Source: CAD feature listing. Evaluate the final solid. Frame: model axes, mm. Face numbers are marked on the shaded views. A direction names the side the tool comes from. Give positions to 0.01 mm unless a question says otherwise; leave off trailing zeros. Write each loop counter-clockwise with the first axis right and the second up, starting at its lowest first coordinate (ties: lowest second). Pieces come first, ordered by that corner, then holes. Notation, with made-up numbers: M -40,-34 L -3,-34 A10 cw -3,-22 Z; hole C -5,-36 d1. An arc over 180 degrees is marked long. Use CSV: the item, a comma, the result in double quotes. Start each with the question number.
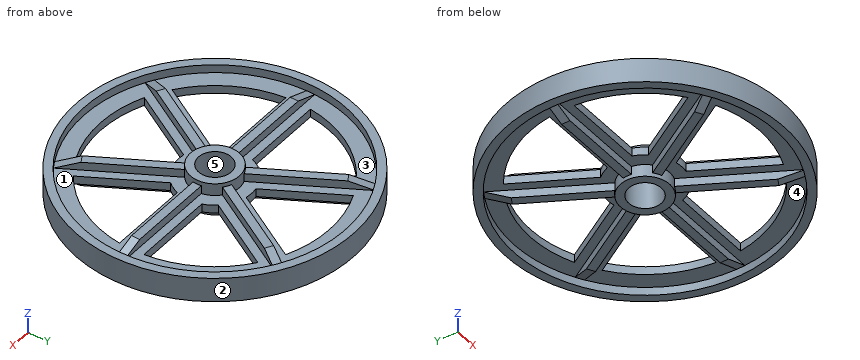
from build123d import *

# Parameters (mm, degrees)
SKETCH1_R           = 15
BOSS_EXTRUDE1_DEPTH = 10
BOSS_EXTRUDE9_DEPTH = 2.5
CIRPATTERN1_COUNT   = 6
CUT_EXTRUDE2_DEPTH  = 5
CIRPATTERN2_COUNT   = 6
SKETCH3_R           = 10
CUT_EXTRUDE3_DEPTH  = 25


with BuildPart() as part:
    # Sketch1 → Boss-Extrude1 (new, symmetric)
    with BuildSketch(Plane.XY):
        Circle(SKETCH1_R)
    extrude(amount=BOSS_EXTRUDE1_DEPTH, both=True)

    # Sketch2 → Revolve1 (revolve)
    with BuildSketch(Plane(origin=(0, 0, 0), x_dir=(0, 0, -1), z_dir=(1, 0, 0)), mode=Mode.PRIVATE) as revolve1_sk:
        Polygon((-2.5, 15), (-2.5, 80), (-7.5, 80), (-7.5, 85), (7.5, 85), (7.5, 80), (2.5, 80), (2.5, 15), align=None)
    revolve(revolve1_sk.sketch.rotate(Axis((0, 0, 0), (0, 0, -1)), 90), axis=Axis((0, 0, 0), (0, 0, -1)))

    # Sketch5 → Boss-Extrude9 (add, symmetric)
    with BuildSketch(Plane(origin=(0, 0, 0), x_dir=(1, 0, 0), z_dir=(0, 1, 0))):
        Polygon((0, -2.5), (-80, -2.5), (-66.262612903, -7.5), (0, -7.5), align=None)
        Polygon((0, 7.5), (-66.262612903, 7.5), (-80, 2.5), (0, 2.5), align=None)
    boss_extrude9 = extrude(amount=BOSS_EXTRUDE9_DEPTH, both=True)

    # CirPattern1: Boss-Extrude9 ×6 about axis
    cirpattern1_axis = Axis((0, 0, 0), (0, 0, 1))
    for i in range(1, CIRPATTERN1_COUNT):
        add(boss_extrude9.rotate(cirpattern1_axis, i * 360 / CIRPATTERN1_COUNT))

    # Sketch6 → Cut-Extrude2 (cut)
    with BuildSketch(Plane.XY.offset(2.5)):
        with BuildLine():
            Line((-17.101792246, 14.621173071), (-41.293717796, 56.522817256))
            ThreePointArc((-41.293717796, 56.522817256), (-60.621778265, 35), (-69.597054535, 7.5))
            Line((-69.597054535, 7.5), (-21.213203436, 7.5))
            ThreePointArc((-21.213203436, 7.5), (-19.485571585, 11.25), (-17.101792246, 14.621173071))
        make_face()
    cut_extrude2 = extrude(amount=-CUT_EXTRUDE2_DEPTH, mode=Mode.SUBTRACT)

    # CirPattern2: Cut-Extrude2 ×6 about axis
    cirpattern2_axis = Axis((0, 0, 0), (0, 0, 1))
    for i in range(1, CIRPATTERN2_COUNT):
        add(cut_extrude2.rotate(cirpattern2_axis, i * 360 / CIRPATTERN2_COUNT), mode=Mode.SUBTRACT)

    # Sketch3 → Cut-Extrude3 (cut)
    with BuildSketch(Plane.XY.offset(10)):
        Circle(SKETCH3_R)
    extrude(amount=-CUT_EXTRUDE3_DEPTH, mode=Mode.SUBTRACT)


solid = part.part
Item 1: Section A-A (x = 0). State how many separate pieces and enclosed holes the cut face has, plus the area to 3 significant figures.
Item 2: Pull-direction query (X, two-part tool) for the marked faces 1 and 2; classes: released by +X, released by -X, zero draft, split by the parting line, or undercut.
Item 3: Section C-C (y = 0). Return the cut outline in (x, z), plus the area to 3 significant figures.
Item 4: Section B-B (z = -5). Return the cut outline in (x, y).
Item 5: Contact query for flat-ended pins moving along their axis: pin 1 Ø6 at (x, z) = (-25, 5.5) entering from -Y; pin 2 Ø2.5 at (x, z) = (49, -6) entering from +Y; pin 3 Ø15 at (x, y) = (-18, -24) entering from +Z. Output: stop coordinate, or through.
Item 6: Section D-D (x = -58). Return the cut outline in (y, z), plus the area to 3 significant figures.
Item 7: Material intervals for probe 1 along Y at (x, z) = (0, 6.3); probe 2 along X at (y, z) = (28, 3); probe 3 along X at (y, z) = (-59, 4.5), sorted ascending.
Item 8: Set-up query: the marked faces 3, 4 and 5. Return all of +Z, -Z, +X, -X, +Y, -Y with unobstructed straight access to the full face (end or side cutting, diameter ignored); none if empty.
Output values:
1,separate pieces,"4"
1,enclosed holes,"0"
1,area,"525 mm2"
2,face 1,"undercut"
2,face 2,"split by the parting line"
3,outline,"M -85,-7.5 L -80,-7.5 L -80,-2.5 L -66.26,-7.5 L -15,-7.5 L -15,-10 L -10,-10 L -10,10 L -15,10 L -15,7.5 L -66.26,7.5 L -80,2.5 L -80,7.5 L -85,7.5 Z; M 10,-10 L 15,-10 L 15,-7.5 L 66.26,-7.5 L 80,-2.5 L 80,-7.5 L 85,-7.5 L 85,7.5 L 80,7.5 L 80,2.5 L 66.26,7.5 L 15,7.5 L 15,10 L 10,10 Z"
3,area,"2,160 mm2"
4,outline,"C 0,0 d170; M -73.13,-2.5 L -14.79,-2.5 A15 ccw -9.56,-11.56 L -38.73,-62.08 L -34.4,-64.58 L -5.23,-14.06 A15 ccw 5.23,-14.06 L 34.4,-64.58 L 38.73,-62.08 L 9.56,-11.56 A15 ccw 14.79,-2.5 L 73.13,-2.5 L 73.13,2.5 L 14.79,2.5 A15 ccw 9.56,11.56 L 38.73,62.08 L 34.4,64.58 L 5.23,14.06 A15 ccw -5.23,14.06 L -34.4,64.58 L -38.73,62.08 L -9.56,11.56 A15 ccw -14.79,2.5 L -73.13,2.5 Z; hole C 0,0 d160; hole C 0,0 d20"
5,pin 1,"stops at y = -82.1"
5,pin 2,"stops at y = 70.32"
5,pin 3,"stops at z = 7.5"
6,outline,"M -62.14,-7.5 L -55.1,-7.5 L -55.1,-2.5 L -39.19,-2.5 L -39.19,2.5 L -55.1,2.5 L -55.1,7.5 L -62.14,7.5 Z; M -7.5,-2.5 L -2.5,-2.5 L -2.5,-7.5 L 2.5,-7.5 L 2.5,-2.5 L 7.5,-2.5 L 7.5,2.5 L 2.5,2.5 L 2.5,7.5 L -2.5,7.5 L -2.5,2.5 L -7.5,2.5 Z; M 39.19,-2.5 L 55.1,-2.5 L 55.1,-7.5 L 62.14,-7.5 L 62.14,7.5 L 55.1,7.5 L 55.1,2.5 L 39.19,2.5 Z"
6,area,"495 mm2"
7,probe 1,"y = -85 to -80, -15 to -10, 10 to 15, 80 to 85"
7,probe 2,"x = -80.26 to -74.94, -19.05 to -13.28, 13.28 to 19.05, 74.94 to 80.26"
7,probe 3,"x = -61.19 to -54.03, -36.95 to -31.18, 31.18 to 36.95, 54.03 to 61.19"
8,face 3,"+Z"
8,face 4,"-Z"
8,face 5,"+Z, -Z"
